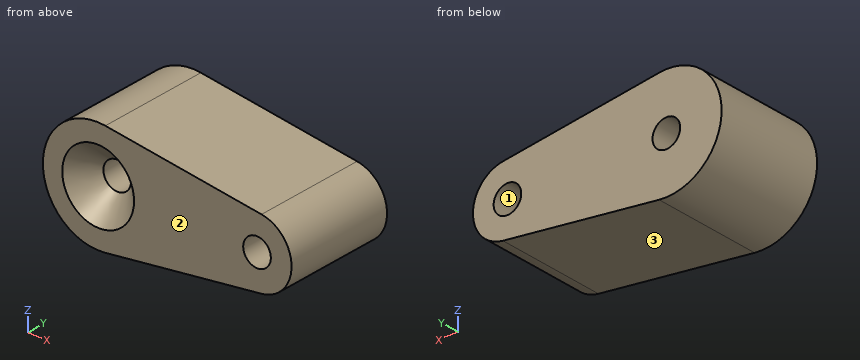
from build123d import *

# Parameters (mm, degrees)
F0_W     = 93.4863612056
F0_H     = 177.5486841798
F0_R     = 7.3874991458
F1_DEPTH = 25.4
F5_R     = 3.175
F6_DEPTH = 25.4
F7_SIZE  = 5.08


# Not quite as in the source:
# - a feature names something its author has since deleted; it is built from what else it names
# - the program builds the solid bodies; features that only make, move or delete a surface that nothing else refers to are left out


with BuildPart() as f1:
    # F0 (on Front) → F1 (new body)
    with BuildSketch(Plane.XZ):
        with Locations((0.2827197313, -1.319359988)):
            Rectangle(F0_W, F0_H)
        Circle(F0_R, mode=Mode.SUBTRACT)
    extrude(amount=F1_DEPTH)


with BuildPart() as f6:
    # F5 (on Front) → F6 (new body)
    with BuildSketch(Plane.XZ):
        with BuildLine():
            ThreePointArc((1.6565217391, -12.5915025207), (9.5479795268, -8.3741320121), (12.7, 0))
            ThreePointArc((12.7, 0), (9.5479795268, 8.3741320121), (1.6565217391, 12.5915025207))
            ThreePointArc((1.6565217391, 12.5915025207), (-12.7, 0), (1.6565217391, -12.5915025207))
        make_face()
        Circle(F5_R, mode=Mode.SUBTRACT)
        with BuildLine():
            ThreePointArc((1.6565217391, 12.5915025207), (9.5479795268, 8.3741320121), (12.7, 0))
            ThreePointArc((12.7, 0), (9.5479795268, -8.3741320121), (1.6565217391, -12.5915025207))
            Line((1.6565217391, -12.5915025207), (37.547826087, -7.8696890754))
            ThreePointArc((37.547826087, -7.8696890754), (28.575, 0), (37.547826087, 7.8696890754))
            Line((37.547826087, 7.8696890754), (1.6565217391, 12.5915025207))
        make_face()
        with BuildLine():
            ThreePointArc((44.45, 0), (42.4799872042, 5.2338325076), (37.547826087, 7.8696890754))
            ThreePointArc((37.547826087, 7.8696890754), (28.575, 0), (37.547826087, -7.8696890754))
            ThreePointArc((37.547826087, -7.8696890754), (42.4799872042, -5.2338325076), (44.45, 0))
        make_face()
        with Locations((36.5125, 0)):
            Circle(F5_R, mode=Mode.SUBTRACT)
    extrude(amount=F6_DEPTH)

    # F7
    f7_edges = [f6.edges().sort_by_distance(p)[0] for p in [
        (-3.175, -25.4, 0),
    ]]
    chamfer(f7_edges, length=F7_SIZE)


solid = f6.part
CAD build for the part. Positions are in the model's coordinates, mm. Face numbers are marked on the shaded views. Round coordinates to 2 decimals unless told otherwise and drop trailing zeros. Loops run counter-clockwise (first coordinate to the right, second up) from the corner with the lowest first, then second, coordinate; pieces in that order, holes last. Notation, with made-up numbers: (-2.75, 59) - (56.25, 59) arc R16 cw to (56.25, 73) - close; hole circle Ø7 at (71.25, -30). An arc over 180 degrees is marked (long way). Put each result on its own line as item: value.
1. Slice it at A-A on z = 0. Give the number of separate pieces and of enclosed holes in the cut face, and give its area (3 significant figures).
Geometry check:
separate pieces: 3
enclosed holes: 0
area: 1,100 mm²
2. Pin check, flat tips, straight feed: P1, Ø3, axis at x = 31.5, y = -13.5, coming from the -Z side; P2, Ø2, axis at x = -6, y = -2.5, coming from the -Z side; P3, Ø4, axis at x = 0, z = 0, coming from the +Y side; P4, Ø1, axis at y = -21, z = -3, coming from the +X side. Stop position of each tip, or through.
Geometry check:
P1: z = -8.86
P2: z = -11.67
P3: through
P4: x = 44.05
3. Slice it at B-B on x = 0. List the corners of the cut face in (y, z) (3 decimals).
Geometry check:
outline: (-25.4, -12.7) - (0, -12.7) - (0, -3.175) - (-20.32, -3.175) - (-25.4, -8.255) - close; (-25.4, 8.255) - (-20.32, 3.175) - (0, 3.175) - (0, 12.7) - (-25.4, 12.7) - close
4. Two-plate mould, pull along X, no slides. Class the marked faces 1, 2 and 3: released by +X, released by -X, zero draft, split by the parting line, or undercut.
Geometry check:
face 1: undercut
face 2: zero draft
face 3: released by +X
5. Wall check: line 1 (Z direction, x = 0, y = -5.25) (3 decimals); line 2 (X direction, y = -15, z = -2.25); line 3 (X direction, y = -6.25, z = -1). Give the ranges that are in metal, low to high.
Geometry check:
line 1: -12.7 to -3.175, 3.175 to 12.7
line 2: -12.5 to -2.24, 2.24 to 34.27, 38.75 to 44.12
line 3: -12.66 to -3.01, 3.01 to 33.5, 39.53 to 44.39
6. Slice it at D-D on x = 36. List the corners of the cut face in (y, z), and give its area (3 significant figures).
Geometry check:
outline: (-25.4, -8.07) - (0, -8.07) - (0, -3.13) - (-25.4, -3.13) - close; (-25.4, 3.13) - (0, 3.13) - (0, 8.07) - (-25.4, 8.07) - close
area: 251 mm²
